Geometry: final body of the model. Coordinates: model frame, mm. Face numbers are marked on the shaded views. Coordinates: 2 decimals unless noted, no trailing zeros. Order: outer loops, then holes, each group sorted by start corner. A loop starts at its lowest first (then second) coordinate and runs counter-clockwise, first axis right, second up. Notation, with made-up numbers: M -28,-24 L -14,-24 A21 ccw -14,-11 Z; hole C 1,31 d6. An arc over 180 degrees is marked long. Use CSV: the item, a comma, the result in double quotes. Start each with the question number.
Q1. Section query C-C, the plane y = 5. Output: boundary loops of the cut face in (x, z).
Q2. Section query D-D, the plane z = -1.7. Output: boundary loops of the cut face in (x, y).
Q3. Mould query, pull axis X, two halves, no side actions, for the marked faces 1, 2 and 3. Classes: +X half, -X half, draft (parallel to the pull), parting line (faces both ways), or undercut.
Q4. Section query B-B, the plane z = -0.8. Output: boundary loops of the cut face in (x, y), and give its area (3 significant figures).
Q5. Ray query, probe 1 along Z at (x, y) = (0, 4.25); probe 2 along X at (y, z) = (4.75, 0.55); probe 3 along Z at (x, y) = (0.4, 12.75). Return the intervals inside material, ascending.
Q6. Section query A-A, the plane x = 0. Output: boundary loops of the cut face in (y, z), and give its area (3 significant figures).
Q7. First-contact query: P1, Ø1.6, axis at x = 0, z = 0, coming from the -Y side; P2, Ø1.5, axis at y = 13, z = -1.5, coming from the +X side. Flat tips, straight axial feed; report the tip coordinate or a pass-through.
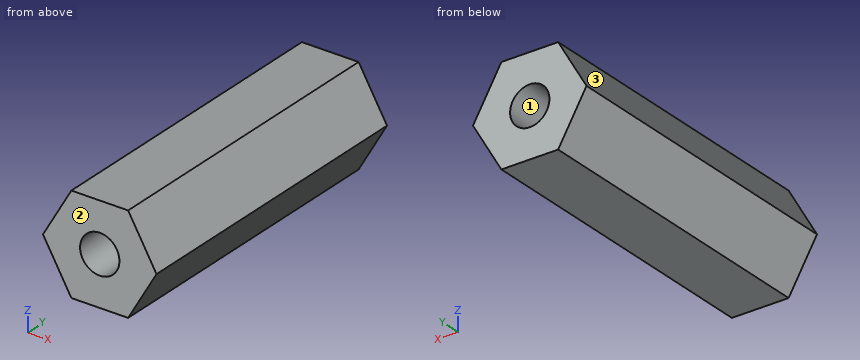
Autodesk Inventor part; units mm, degrees
ref_plane "YZ Plane" through (0, 0, 0) normal (1, 0, 0) x (0, 1, 0)
ref_plane "XZ Plane" through (0, 0, 0) normal (0, 1, 0) x (-1, 0, 0)
ref_plane "XY Plane" through (0, 0, 0) normal (0, 0, 1) x (1, 0, 0)
sketch "Эскиз1" plane through (0, 0, 0) normal (0, 1, 0) x (-1, 0, 0)
  line L0 (1.4434, 2.5) -> (2.8868, 0)
  line L1 (2.8868, 0) -> (1.4434, -2.5)
  line L2 (1.4434, -2.5) -> (-1.4434, -2.5)
  line L3 (-1.4434, -2.5) -> (-2.8868, 0)
  line L4 (-2.8868, 0) -> (-1.4434, 2.5)
  line L5 (-1.4434, 2.5) -> (1.4434, 2.5)
  point P0 (0, 0)
  point P1 (0, 0)
  dimension "d0" = 5
extrude "Выдавливание1" add sketch "Эскиз1" along normal blind 15.9
sketch "Эскиз2" plane through (0, 15.9, 0) normal (0, 1, 0) x (1, 0, 0)
  line L0 (1.4434, 2.5) -> (-1.4434, 2.5)
  line L1 (-1.4434, 2.5) -> (-2.8868, 0)
  line L2 (-2.8868, 0) -> (-1.4434, -2.5)
  line L3 (-1.4434, -2.5) -> (1.4434, -2.5)
  line L4 (1.4434, -2.5) -> (2.8868, 0)
  line L5 (2.8868, 0) -> (1.4434, 2.5)
  point P0 (0, 0)
hole "Отверстие1" at (0, 15.9, 0) direction (0, -1, 0) diameter 2 end through all
properties part number "Проставка для стойки RPLIDAR"
Responses:
1,outline,"M -2.89,0 L -1.44,-2.5 L 1.44,-2.5 L 2.89,0 L 1.44,2.5 L -1.44,2.5 Z; hole C 0,0 d2"
2,outline,"M -1.91,0 L 1.91,0 L 1.91,15.9 L -1.91,15.9 Z"
3,face 1,"undercut"
3,face 2,"draft"
3,face 3,"-X half"
4,outline,"M -2.42,0 L -0.6,0 L -0.6,15.9 L -2.42,15.9 Z; M 0.6,0 L 2.42,0 L 2.42,15.9 L 0.6,15.9 Z"
4,area,"58.0 mm²"
5,probe 1,"z = -2.5 to -1, 1 to 2.5"
5,probe 2,"x = -2.57 to -0.84, 0.84 to 2.57"
5,probe 3,"z = -2.5 to -0.92, 0.92 to 2.5"
6,outline,"M 0,-2.5 L 15.9,-2.5 L 15.9,-1 L 0,-1 Z; M 0,1 L 15.9,1 L 15.9,2.5 L 0,2.5 Z"
6,area,"47.7 mm²"
7,P1,"passes through"
7,P2,"stops at x = 2.45"
